```python
from build123d import *

# Parameters (mm, degrees)
EXTRUDE070_DEPTH                     = 5
EXTRUDE070_ONTO_SKETCH267_ROLL_ANGLE = 90
SKETCH268_AS_DRAWN_R                 = 1
EXTRUDE069_DEPTH                     = 10
EXTRUDE069_ONTO_SKETCH268_ROLL_ANGLE = 90
EXTRUDE071_DEPTH                     = 1
EXTRUDE071_ONTO_SKETCH266_ROLL_ANGLE = 90


with BuildPart() as extrude070:
    # Sketch267 as drawn → Extrude070 (new)
    with BuildSketch(Plane.XY):
        with BuildLine():
            ThreePointArc((8.500012, 10), (5.490931, 6.990186), (8.501267, 3.981628))
            ThreePointArc((8.501267, 3.981628), (9.735803, 4.24621), (10.754109, 4.992623))
            ThreePointArc((11.751661, 5.997636), (11.044132, 5.702333), (10.754109, 4.992623))
            Line((11.751661, 5.997636), (12.000229, 5.997636))
            ThreePointArc((12.999313, 4.999389), (12.706459, 5.705374), (12.000229, 5.997636))
            Line((12.999313, 4.999389), (15.5, 5))
            Line((15.5, 5), (15.5, 9))
            Line((13, 9), (15.5, 9))
            ThreePointArc((12, 8), (12.707107, 8.292893), (13, 9))
            Line((11.75, 8), (12, 8))
            ThreePointArc((10.75, 9), (11.042893, 8.292893), (11.75, 8))
            ThreePointArc((10.75, 9), (9.731212, 9.738962), (8.500012, 10))
        make_face()
    extrude(amount=-EXTRUDE070_DEPTH)


with BuildPart() as extrude070_1:
    # Extrude070 onto Sketch267 roll: moved
    add(extrude070.part.rotate(Axis((0, 0, 0), (1, 0, 0)), EXTRUDE070_ONTO_SKETCH267_ROLL_ANGLE))


with BuildPart() as extrude070_2:
    # Extrude070 onto Sketch267 placement: moved
    add(extrude070_1.part.moved(Location((0, 3, 0))))


with BuildPart() as extrude069:
    # Sketch268 as drawn → Extrude069 (new)
    with BuildSketch(Plane.XY):
        with Locations((8.5, 12)):
            Circle(SKETCH268_AS_DRAWN_R)
    extrude(amount=-EXTRUDE069_DEPTH)


with BuildPart() as extrude069_1:
    # Extrude069 onto Sketch268 roll: moved
    add(extrude069.part.rotate(Axis((0, 0, 0), (1, 0, 0)), EXTRUDE069_ONTO_SKETCH268_ROLL_ANGLE))


with BuildPart() as extrude069_2:
    # Extrude069 onto Sketch268 placement: moved
    add(extrude069_1.part.moved(Location((0, 4, 0))))


with BuildPart() as extrude069_3:
    # Extrude069 placement: moved
    add(extrude069_2.part.moved(Location((0, -2, 0))))


with BuildPart() as cut042:
    # Sketch266 as drawn → Extrude071 (new)
    with BuildSketch(Plane.XY):
        with BuildLine():
            Line((0, 1), (0, 10))
            ThreePointArc((2, 12), (0.585786, 11.414214), (0, 10))
            Line((2, 12), (6, 12))
            ThreePointArc((6, 12), (6.707107, 12.292893), (7, 13))
            ThreePointArc((10, 13.000001), (8.5, 13.802776), (7, 13))
            ThreePointArc((10, 13.000001), (10.292893, 12.292893), (11, 12))
            Line((12, 12), (11, 12))
            ThreePointArc((13, 11), (12.707107, 11.707107), (12, 12))
            Line((13, 1), (13, 11))
            Line((0, 1), (13, 1))
        make_face()
    extrude(amount=-EXTRUDE071_DEPTH)


with BuildPart() as cut042_1:
    # Extrude071 onto Sketch266 roll: moved
    add(cut042.part.rotate(Axis((0, 0, 0), (1, 0, 0)), EXTRUDE071_ONTO_SKETCH266_ROLL_ANGLE))


with BuildPart() as cut042_2:
    # Extrude071 onto Sketch266 placement: moved
    add(cut042_1.part.moved(Location((0, 6, 0))))

    # Cut041: cut Extrude069
    add(extrude069_3.part, mode=Mode.SUBTRACT)

    # Cut042: cut Extrude070
    add(extrude070_2.part, mode=Mode.SUBTRACT)


solid = cut042_2.part
```
CAD build for the part. Positions are in the model's coordinates, mm. A direction names the side the tool comes from. Give positions to 0.01 mm unless a question says otherwise; leave off trailing zeros. Loops run counter-clockwise (first coordinate to the right, second up) from the corner with the lowest first, then second, coordinate; pieces in that order, holes last. Notation, with made-up numbers: M -23.75,54.5 L 20.25,54.5 A20 ccw 20.25,69.5 Z; hole C -15.5,-5 d8. An arc over 180 degrees is marked long. Use one line per item in the form item = value.
Item 1: Drill centre lines: probe 1 along Z at (x, y) = (8.5, 6.3); probe 2 along Z at (x, y) = (11.75, 6.4); probe 3 along Z at (x, y) = (6, 6.5). Where is each one in solid material? Low to high. Write a range as from..to.
Determined:
probe_1 = 1..3.98, 10..11, 13..13.8
probe_2 = 1..6, 8..12
probe_3 = 1..5.32, 8.67..12
Item 2: Slice it at A-A (x = 5.75). List the corners of the cut face in (y, z).
Determined:
outline = M 6,1 L 7,1 L 7,5.77 L 6,5.77 Z; M 6,8.21 L 7,8.21 L 7,12 L 6,12 Z
Item 3: Two-plate mould, pull along Z, no slides. Class faces 1 (the face through (11.5, 6.5, 12)), 2 (the face through (13, 6.5, 3)), 3 (the face through (5.49, 6.49, 7.06)): pulls with the +Z half, pulls with the -Z half, needs draft (parallel to the pull), parting line crosses it, or undercut.
Determined:
face_1 = pulls with the +Z half
face_2 = needs draft
face_3 = undercut
Item 4: Slice it at D-D (z = 7.75). List the corners of the cut face in (x, y).
Determined:
outline = M 0,6 L 5.59,6 L 5.59,7 L 0,7 Z
Item 5: Which spindle directions (+Z, -Z, +X, -X, +Y, -Y) get a long thin tool onto all of the face, cutting with end or side? Do faces 4 (the face through (4, 6.5, 12)), 5 (the face through (12.699, 6.493, 8.285)), 6 (the face through (11.05, 6.49, 5.71)). Say none if no direction does.
Determined:
face_4 = +Z, -X, +Y, -Y
face_5 = +X, +Y, -Y
face_6 = +Y, -Y
Item 6: Slice it at C-C (z = 12.25). List the corners of the cut face in (x, y).
Determined:
outline = M 6.66,6 L 7.53,6 L 7.53,7 L 6.66,7 Z; M 9.47,6 L 10.34,6 L 10.34,7 L 9.47,7 Z
